```python
from build123d import *
from build123d.topology import SkipClean

# Parameters (mm, degrees)
SKETCH3_R           = 14.9225
BOSS_EXTRUDE1_DEPTH = 12.7
SKETCH11_R          = 2.38125
CUT_EXTRUDE3_DEPTH  = 6.35
SKETCH12_R          = 7.874
SKETCH12_R_2        = 6.35
CUT_EXTRUDE4_DEPTH  = 2.54
THREAD1_PITCH       = 1.5875
CUT_EXTRUDE5_START  = -6.35
SKETCH13_R          = 2.38125
CUT_EXTRUDE5_DEPTH  = 6.35
CUT_EXTRUDE6_START  = -6.35
SKETCH14_R          = 14.9225
CUT_EXTRUDE6_DEPTH  = 6.35


with BuildPart() as part:
    # Sketch3 → Boss-Extrude1 (new body)
    with BuildSketch(Plane.XY):
        with Locations((8.347593151, 27.723781851)):
            Circle(SKETCH3_R)
    extrude(amount=-BOSS_EXTRUDE1_DEPTH)

    # Sketch11 → Cut-Extrude3 (cut)
    with BuildSketch(Plane.XY):
        with Locations((8.347593151, 27.723781851)):
            Circle(SKETCH11_R)
    extrude(amount=-CUT_EXTRUDE3_DEPTH, mode=Mode.SUBTRACT)

    # Sketch12 → Cut-Extrude4 (cut)
    with BuildSketch(Plane.XY):
        with Locations((8.347593151, 27.723781851)):
            Circle(SKETCH12_R)
        with Locations((8.347593151, 27.723781851)):
            Circle(SKETCH12_R_2, mode=Mode.SUBTRACT)
    extrude(amount=-CUT_EXTRUDE4_DEPTH, mode=Mode.SUBTRACT)

    # Thread1: the profile of Thread Profile1 profile screwed along a right-hand helix of 4.8 turns, 8 arcs to a turn; built about Z, then put on its axis
    thread1_z = Axis((0, 0, 0), (0, 0, 1))
    thread1_corners = [(14.9228, 0, -0.000173205), (14.9228, 0, 0.694704453), (14.492870212, 0, 0.446484374), (14.492870212, 0, 0.248046874)]
    with BuildLine(mode=Mode.PRIVATE) as thread1_profile:
        Line(thread1_corners[0], thread1_corners[1])
        Line(thread1_corners[1], thread1_corners[2])
        Line(thread1_corners[2], thread1_corners[3])
        Line(thread1_corners[3], thread1_corners[0])
    thread1_cap = Face(thread1_profile.wire())
    thread1_turn_angles = [0, 22.5, 45, 67.5, 90, 112.5, 135, 157.5, 180, 202.5, 225, 247.5, 270, 292.5, 315, 337.5, 360]
    thread1_turn_weights = [1, 0.9238795325112867, 1, 0.9238795325112867, 1, 0.9238795325112867, 1, 0.9238795325112867, 1, 0.9238795325112867, 1, 0.9238795325112867, 1, 0.9238795325112867, 1, 0.9238795325112867, 1]
    thread1_turn_rails = [Edge.make_bspline([Vector(p[0], p[1], 0).rotate(thread1_z, thread1_turn_angles[k]) / thread1_turn_weights[k] + Vector(0, 0, p[2] + THREAD1_PITCH * thread1_turn_angles[k] / 360) for k in range(17)], [0, 0, 0, 1, 1, 2, 2, 3, 3, 4, 4, 5, 5, 6, 6, 7, 7, 8, 8, 8], 2, thread1_turn_weights) for p in thread1_corners]
    thread1_turn_sides = [Face.make_surface_from_curves(thread1_turn_rails[p[0]], thread1_turn_rails[p[1]]) for p in [(0, 1), (1, 2), (2, 3), (3, 0)]]
    thread1_last_angles = [1440, 1462.5, 1485, 1507.5, 1530, 1552.5, 1575, 1597.5, 1620, 1642.5, 1665, 1687.5, 1710, 1719, 1728]
    thread1_last_weights = [1, 0.9238795325112867, 1, 0.9238795325112867, 1, 0.9238795325112867, 1, 0.9238795325112867, 1, 0.9238795325112867, 1, 0.9238795325112867, 1, 0.9876883405951378, 1]
    thread1_last_rails = [Edge.make_bspline([Vector(p[0], p[1], 0).rotate(thread1_z, thread1_last_angles[k]) / thread1_last_weights[k] + Vector(0, 0, p[2] + THREAD1_PITCH * thread1_last_angles[k] / 360) for k in range(15)], [0, 0, 0, 1, 1, 2, 2, 3, 3, 4, 4, 5, 5, 6, 6, 7, 7, 7], 2, thread1_last_weights) for p in thread1_corners]
    thread1_last_sides = [Face.make_surface_from_curves(thread1_last_rails[p[0]], thread1_last_rails[p[1]]) for p in [(0, 1), (1, 2), (2, 3), (3, 0)]]
    thread1 = Plane(origin=(8.347593151, 27.723781851, 0.79375), x_dir=(-1, 0, 0), z_dir=(0, 0, -1)) * Solid(Shell([*[p.moved(Location((0, 0, THREAD1_PITCH * i))) for i in range(4) for p in thread1_turn_sides], *thread1_last_sides, thread1_cap, thread1_cap.rotate(thread1_z, 1728).moved(Location((0, 0, THREAD1_PITCH * 1728 / 360)))]))
    add(thread1, mode=Mode.SUBTRACT)

    # Sketch13 → Cut-Extrude5 (cut)
    with BuildSketch(Plane(origin=(0, 0, -12.7), x_dir=(-1, 0, 0), z_dir=(0, 0, -1)).offset(CUT_EXTRUDE5_START)):
        with Locations(Location((-8.347593151, 27.723781851, 0), (0, 0, 180))):
            Circle(SKETCH13_R)
    extrude(amount=CUT_EXTRUDE5_DEPTH, mode=Mode.SUBTRACT)

    # Sketch14 → Cut-Extrude6 (cut)
    with SkipClean():  # the faces are left unmerged after this step: merging them gives an invalid solid
        with BuildSketch(Plane(origin=(0, 0, -12.7), x_dir=(-1, 0, 0), z_dir=(0, 0, -1)).offset(CUT_EXTRUDE6_START)):
            with Locations((-8.347593151, 27.723781851)):
                Circle(SKETCH14_R)
            Polygon((1.186658464, 22.240576024), (1.168128197, 33.239083042), (-8.366123418, 38.722288869), (-17.881844766, 33.206987678), (-17.863314499, 22.20848066), (-8.329062884, 16.725274833), align=None, mode=Mode.SUBTRACT)
        extrude(amount=CUT_EXTRUDE6_DEPTH, mode=Mode.SUBTRACT)
    add(part.part.scale(1), mode=Mode.REPLACE)  # the faces are merged on a copy


solid = part.part
```
Check sheet for the modelled part. Datum: model origin and axes. Units: mm. A direction names the side the tool comes from. Round coordinates to 2 decimals unless told otherwise and drop trailing zeros. Write each loop counter-clockwise with the first axis right and the second up, starting at its lowest first coordinate (ties: lowest second). Pieces come first, ordered by that corner, then holes. Notation, with made-up numbers: M -21.5,39 L 18.5,39 A29 ccw 18.5,72 Z; hole C -1.75,45.25 d8. An arc over 180 degrees is marked long. Write item = value, one per line. Start each with the question number.
1. Release check for a two-part mould opening along X. For faces 6 (the cylindrical face through (7.52, 34.02, -1.25)), 7 (the flat face through (3.53, 35.94, -9.48)), 8 (the flat face through (8, 25, 0)) record: pulls with the +X half, pulls with the -X half, needs draft (parallel to the pull), parting line crosses it, or undercut.
2. Gauge pin test, flat ends, axial feed: pin 1 (3 mm diameter, centred on x = 8.35, y = 27.72, fed in from +Z); pin 2 (6 mm diameter, centred on y = 22, z = -10, fed in from +X); pin 3 (4 mm diameter, centred on y = 18, z = -10, fed in from -X); pin 4 (4 mm diameter, centred on y = 37.5, z = -4, fed in from -X). Record the tip position at first contact, or that the pin passes through.
3. Tool access check on faces 1 (the cylindrical face through (11.981, 20.738, -1.252)), 2 (the flat face through (3.638, 19.444, -9.481)), 3 (the flat face through (13.163, 19.505, -9.481)), 4 (the flat face through (13.06, 36, -9.48)), 5 (the flat face through (-1.4, 27.7, -6.35)). Record the directions out of +Z, -Z, +X, -X, +Y, -Y that give a thin tool (end or side, any length) a straight path to the whole face; none if there is none.
4. Scan lines: line 1 (X direction, y = 31, z = -1.75); line 2 (Z direction, x = 18.5, y = 25.5); line 3 (X direction, y = 27.5, z = -9). Record each from-to range of solid material in increasing order. Write a range as [from, to].
5. Section check A-A, the plane z = -9. Record the cut outline in (x, y), then the cut area to 3 significant figures.
Results found:
q1.face_6 = undercut
q1.face_7 = pulls with the -X half
q1.face_8 = needs draft
q2.pin_1 = through
q2.pin_2 = 17.87
q2.pin_3 = 2.68
q2.pin_4 = -4.39
q3.face_1 = +Z
q3.face_2 = -Z, -X, -Y
q3.face_3 = -Z, +X, -Y
q3.face_4 = -Z, +X, +Y
q3.face_5 = -Z
q4.line_1 = [-6.21, 1.19], [2.91, 13.79], [15.51, 22.52]
q4.line_2 = [-6.35, 0]
q4.line_3 = [-1.18, 5.98], [10.72, 17.87]
q5.outline = M -1.19,22.24 L 8.33,16.73 L 17.86,22.21 L 17.88,33.21 L 8.37,38.72 L -1.17,33.24 Z; hole C 8.35,27.72 d4.76
q5.area = 296 mm^2
